```python
from build123d import *

# Parameters (mm, degrees)
F0_W     = 1000
F0_H     = 30
F1_DEPTH = 30
F3_DEPTH = 2027
F5_DEPTH = 2087


with BuildPart() as f1:
    # F0 (on Front) → F1 (new body)
    with BuildSketch(Plane.XZ):
        with Locations((-500, 24.806101)):
            Rectangle(F0_W, F0_H)
    extrude(amount=F1_DEPTH)

    # F2 (on face) → F3 (cut)
    with BuildSketch(Plane(origin=(-1000, 0, 0), x_dir=(0, -1, 0), z_dir=(-1, 0, 0))):
        Polygon((20.216802, 23.715444), (16.909165, 39.806101), (6.909165, 39.806101), (10.394015, 20.198643), align=None)
    extrude(amount=-F3_DEPTH, mode=Mode.SUBTRACT)

    # F4 (on face) → F5 (cut)
    with BuildSketch(Plane(origin=(-1000, 0, 0), x_dir=(0, -1, 0), z_dir=(-1, 0, 0))):
        Polygon((30, 39.806101), (22.5, 49.806101), (30, 24.806101), align=None)
    extrude(amount=-F5_DEPTH, mode=Mode.SUBTRACT)


solid = f1.part
```
For this review, take the finished solid that the model builds, in its own axes (mm). Round coordinates to 2 decimals unless told otherwise and drop trailing zeros. Loops run counter-clockwise (first coordinate to the right, second up) from the corner with the lowest first, then second, coordinate; pieces in that order, holes last.
(1) Mouldability with a two-part tool opening along Z and no side actions: class faces 1 (the flat face through (-507, -8.627, 30.14)), 2 (the flat face through (-507, 0, 25)), 3 (the flat face through (-507, -18.586, 31.648)) as released by +Z, released by -Z, zero draft, split by the parting line, or undercut.
Returned:
face 1: released by +Z
face 2: zero draft
face 3: undercut
(2) Wall thickness on line 1 along Y through (x, z) = (-100, 39.5); line 2 along Y through (x, z) = (-578.5, 33.5); line 3 along Z through (x, y) = (-757, -11): over which ranges is each line inside the solid? List them lowest first.
Returned:
line 1: y = -25.59 to -16.97, -6.96 to 0
line 2: y = -27.39 to -18.21, -8.03 to 0
line 3: z = 9.81 to 20.42
(3) Clearance check with a flat-ended pin moving along its axis: P1, Ø1.5, axis at x = -688.5, z = 34, coming from the -Y side. State where the tip first meets the part, or that it passes through.
Returned:
P1: stops at y = -27.47
(4) We need section A-A (z = 34). Give the boundary of the cut face in (x, y), plus the area to 3 significant figures.
Returned:
outline: (-1000, -27.24) - (0, -27.24) - (0, -18.1) - (-1000, -18.1) - close; (-1000, -7.94) - (0, -7.94) - (0, 0) - (-1000, 0) - close
area: 17,100 mm2
(5) We need section B-B (x = -87). Give the boundary of the cut face in (y, z), plus the area to 3 significant figures.
Returned:
outline: (-30, 9.81) - (0, 9.81) - (0, 39.81) - (-6.91, 39.81) - (-10.39, 20.2) - (-20.22, 23.72) - (-16.91, 39.81) - (-25.5, 39.81) - (-30, 24.81) - close
area: 683 mm2
